Verification items for the finished model (mm, model axes). A direction names the side the tool comes from. Coordinates: 2 decimals unless noted, no trailing zeros. Order: outer loops, then holes, each group sorted by start corner. A loop starts at its lowest first (then second) coordinate and runs counter-clockwise, first axis right, second up. Notation, with made-up numbers: (27.5, 46.5) -> (58.5, 46.5) arc R15 cw to (58.5, 69.5) -> close; hole circle Ø7 at (50.25, 16). An arc over 180 degrees is marked (long way). Write item = value, one per line. Start each with the question number.
1. Cross-section at A-A on x = 4.25. Record the cut outline in (y, z).
2. Go/stop test with flat-tipped pins: P1, Ø7.5, axis at y = 17.5, z = 17.5, coming from the -X side; P2, Ø1, axis at x = 6.5, z = 25, coming from the +Y side; P3, Ø1, axis at x = -1.5, y = 16.5, coming from the +Z side; P4, Ø1.6, axis at x = -1, y = 17.5, coming from the -Z side. Record where each tip stops, or that it passes through.
3. Cross-section at B-B on y = 4. Record the cut outline in (x, z), plus the area to 3 significant figures.
4. Set-up check for faces 1 (the flat face through (-1, 16, 27.05)), 2 (the flat face through (4, 18, -1)), 3 (the flat face through (4, 15, -1)), 4 (the flat face through (11, 15, 3)): record each of +Z, -Z, +X, -X, +Y, -Y from which the full face is reachable in a straight line by a thin tool's end or side.
5. Release check for a two-part mould opening along Y. For faces 5 (the cylindrical face through (16.4, 12.07, 1.52)), 6 (the flat face through (2, 16, 14.35)), 7 (the flat face through (3.986, 12.844, 4.846)), 8 (the flat face through (15, 18, -1)) record: +Y half, -Y half, draft (parallel to the pull), parting line (faces both ways), or undercut.
6. Thickness scan on line 1 along Y through (x, z) = (-0.75, 18.5); line 2 along Y through (x, z) = (0.15, 18.45); line 3 along Z through (x, y) = (1.85, 4). Record the ranges inside material, lowest first. Write a range as from..to.
7. Cross-section at D-D on x = 11. Record the cut outline in (y, z).
8. Cross-section at C-C on z = 29. Record the cut outline in (x, y).
from build123d import *

# Parameters (mm, degrees)
SKETCH002_W     = 10
SKETCH002_H     = 3
PAD004_DEPTH    = 12
SKETCH006_R     = 1.6
POCKET_DEPTH    = 5
SKETCH004_W     = 3
SKETCH004_H     = 9
SKETCH004_H_2   = 2
PAD002_DEPTH    = 1.2
SKETCH005_R     = 7.55
PAD001_DEPTH    = 2
SKETCH_W        = 28
SKETCH_H        = 33
SKETCH_R        = 1.1
SKETCH_W_2      = 8.3
SKETCH_H_2      = 8.3
PAD_DEPTH       = 3
SKETCH001_R     = 2.1
SKETCH001_R_2   = 1.1
SKETCH001_R_3   = 2.71418
PAD003_DEPTH    = 2
FILLET_R        = 2
FILLET001_R     = 2
FILLET002_R     = 0.5
SKETCH007_R     = 7.5
POCKET001_DEPTH = 0.5


with BuildPart() as pocket:
    # Sketch002 → Pad004 (new body)
    with BuildSketch(Plane.YZ.offset(5)):
        with Locations((16.5, 1.5)):
            Rectangle(SKETCH002_W, SKETCH002_H)
    extrude(amount=PAD004_DEPTH)

    # Sketch006 → Pocket (cut)
    with BuildSketch(Plane(origin=(5, 0, 3), x_dir=(0, -1, 0), z_dir=(0, 0, 1))):
        with Locations((-16.5, 7)):
            Circle(SKETCH006_R)
    extrude(amount=-POCKET_DEPTH, mode=Mode.SUBTRACT)


with BuildPart() as pad002:
    # Sketch004 → Pad002 (new body)
    with BuildSketch(Plane.YX):
        with Locations((16.5, 4.5)):
            Rectangle(SKETCH004_W, SKETCH004_H)
        with Locations((16.5, 15)):
            Rectangle(SKETCH004_W, SKETCH004_H_2)
    extrude(amount=PAD002_DEPTH)


with BuildPart() as pad001:
    # Sketch005 → Pad001 (new body)
    with BuildSketch(Plane(origin=(0, 0, 0), x_dir=(0, 1, 0), z_dir=(-1, 0, 0))):
        with BuildLine():
            ThreePointArc((12.4754, -9.95), (7.050137, -18.5), (12.4754, -27.05))
            Line((12.4754, -27.05), (20.5246, -27.05))
            ThreePointArc((20.5246, -27.05), (25.949863, -18.5), (20.5246, -9.95))
            Line((12.4754, -9.95), (20.5246, -9.95))
        make_face()
        with Locations((16.5, -18.5)):
            Circle(SKETCH005_R, mode=Mode.SUBTRACT)
    extrude(amount=PAD001_DEPTH)


with BuildPart() as pad:
    # Sketch → Pad (new body)
    with BuildSketch(Plane.YZ):
        with Locations((14, 16.5)):
            Rectangle(SKETCH_W, SKETCH_H)
        with Locations((16.5, 29)):
            Circle(SKETCH_R, mode=Mode.SUBTRACT)
        with Locations((4, 29)):
            Circle(SKETCH_R, mode=Mode.SUBTRACT)
        with Locations((4, 8)):
            Circle(SKETCH_R, mode=Mode.SUBTRACT)
        with Locations((16.5, 8)):
            Circle(SKETCH_R, mode=Mode.SUBTRACT)
        with Locations((16.5, 18.5)):
            Rectangle(SKETCH_W_2, SKETCH_H_2, mode=Mode.SUBTRACT)
    extrude(amount=PAD_DEPTH)


with BuildPart() as pocket001:
    # Sketch001 → Pad003 (new body)
    with BuildSketch(Plane.YZ.offset(3)):
        with Locations((4, 8)):
            Circle(SKETCH001_R)
        with Locations((4, 8)):
            Circle(SKETCH001_R_2, mode=Mode.SUBTRACT)
        with Locations((4, 29)):
            Circle(SKETCH001_R_3)
        with Locations((4, 29)):
            Circle(SKETCH001_R_2, mode=Mode.SUBTRACT)
        with Locations((16.5, 29)):
            Circle(SKETCH001_R_3)
        with Locations((16.5, 29)):
            Circle(SKETCH001_R_2, mode=Mode.SUBTRACT)
        with BuildLine():
            ThreePointArc((16.5, 10.71418), (14.148967, 9.356252), (14.15042, 6.641234))
            Line((14.15042, 6.641234), (11.5, 3))
            Line((11.5, 0), (11.5, 3))
            Line((21.5, 0), (11.5, 0))
            Line((21.5, 3), (21.5, 0))
            Line((18.84958, 6.641234), (21.5, 3))
            ThreePointArc((18.84958, 6.641234), (18.851033, 9.356252), (16.5, 10.71418))
        make_face()
        with Locations((16.5, 8)):
            Circle(SKETCH001_R_2, mode=Mode.SUBTRACT)
    extrude(amount=PAD003_DEPTH)

    # Fusion: union Pocket, Pad002, Pad001, Pad
    add(pocket.part)
    add(pad002.part)
    add(pad001.part)
    add(pad.part)

    # Fillet
    fillet_edges = [pocket001.edges().sort_by_distance(p)[0] for p in [
        (1.5, 28, 33),
        (1.5, 0, 33),
        (1.5, 0, 0),
        (1.5, 28, 0),
    ]]
    fillet(fillet_edges, radius=FILLET_R)

    # Fillet001
    fillet001_edges = [pocket001.edges().sort_by_distance(p)[0] for p in [
        (17, 11.5, 1.5),
        (17, 21.5, 1.5),
    ]]
    fillet(fillet001_edges, radius=FILLET001_R)

    # Fillet002
    fillet002_edges = [pocket001.edges().sort_by_distance(p)[0] for p in [
        (9, 16.5, -1.2),
        (14, 16.5, -1.2),
        (16, 16.5, -1.2),
        (0, 16.5, -1.2),
    ]]
    fillet(fillet002_edges, radius=FILLET002_R)

    # Sketch007 → Pocket001 (cut)
    with BuildSketch(Plane(origin=(0, 0, 0), x_dir=(0, -1, 0), z_dir=(-1, 0, 0))):
        with Locations((-16.5246, 18.45)):
            Circle(SKETCH007_R)
    extrude(amount=-POCKET001_DEPTH, mode=Mode.SUBTRACT)


solid = pocket001.part
Worked out:
q1.outline = circle Ø5.43 at (4, 29); circle Ø4.2 at (4, 8); (11.5, 0) -> (15, 0) -> (15, -1.2) -> (18, -1.2) -> (18, 0) -> (21.5, 0) -> (21.5, 3) -> (18.85, 6.64) arc R2.71 ccw to (16.5, 10.71) arc R2.71 ccw to (14.15, 6.64) -> (11.5, 3) -> close; circle Ø5.43 at (16.5, 29); hole circle Ø2.2 at (4, 8); hole circle Ø2.2 at (4, 29); hole circle Ø2.2 at (16.5, 8); hole circle Ø2.2 at (16.5, 29)
q2.P1 = 0.5
q2.P2 = through
q2.P3 = 27.05
q2.P4 = 9.95
q3.outline = (0, 0) -> (3, 0) -> (3, 5.9) -> (5, 5.9) -> (5, 6.9) -> (0, 6.9) -> close; (0, 9.1) -> (5, 9.1) -> (5, 10.1) -> (3, 10.1) -> (3, 26.29) -> (5, 26.29) -> (5, 27.9) -> (0, 27.9) -> close; (0, 30.1) -> (5, 30.1) -> (5, 31.71) -> (3, 31.71) -> (3, 33) -> (0, 33) -> close
q3.area = 96.3 mm²
q4.face_1 = +Z, -X, +Y, -Y
q4.face_2 = -Z, +X, -X, +Y
q4.face_3 = -Z, +X, -X, -Y
q4.face_4 = +Z, +X, +Y, -Y
q5.face_5 = -Y half
q5.face_6 = undercut
q5.face_7 = undercut
q5.face_8 = +Y half
q6.line_1 = 7.05..8.95, 24.05..25.95
q6.line_2 = 0..9.02, 24.02..28
q6.line_3 = 0..6.9, 9.1..27.9, 30.1..33
q7.outline = (11.5, 0) -> (15.25, 0) -> (15.25, 3) -> (11.5, 3) -> close; (17.75, 0) -> (21.5, 0) -> (21.5, 3) -> (17.75, 3) -> close
q8.outline = (0, 0) -> (3, 0) -> (3, 1.29) -> (5, 1.29) -> (5, 2.9) -> (0, 2.9) -> close; (0, 5.1) -> (5, 5.1) -> (5, 6.71) -> (3, 6.71) -> (3, 13.79) -> (5, 13.79) -> (5, 15.4) -> (0, 15.4) -> close; (0, 17.6) -> (5, 17.6) -> (5, 19.21) -> (3, 19.21) -> (3, 28) -> (0, 28) -> close
